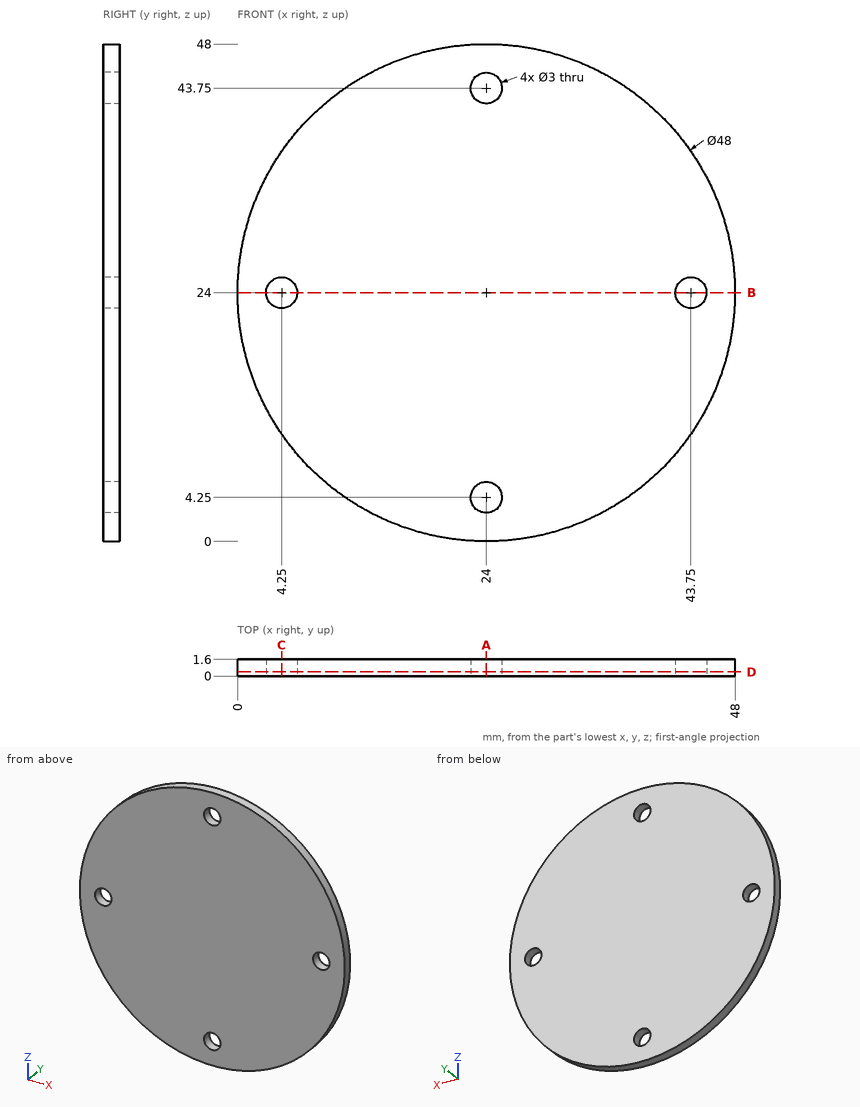
Source: three-view drawing plus pictorial views. Frame: mm from the lowest corner of the part. Round coordinates to 2 decimals unless told otherwise and drop trailing zeros. Write each loop counter-clockwise with the first axis right and the second up, starting at its lowest first coordinate (ties: lowest second). Pieces come first, ordered by that corner, then holes. Notation, with made-up numbers: M -29.5,-38 L 23.5,-38 A18 ccw 23.5,-24 Z; hole C 50,1.25 d2. An arc over 180 degrees is marked long. One line per item, written item: value. Start each with the question number.
Item 1: Section query D-D (y = 0.4). Return the cut outline in (x, z).
Item 2: Section query A-A (x = 24). Return the cut outline in (y, z), plus the area to 3 significant figures.
Item 3: Pin query (flat end, axial travel): pin 1 (2.5 mm diameter, centred on x = 24, z = 4.25, fed in from -Y). Return the tip coordinate at first contact, or that it passes through.
Item 4: Ray query, L1, parallel to X at y = 1.05, z = 24; L2, parallel to X at y = 0.7, z = 23; L3, parallel to Z at x = 45, y = 1.5. Return the intervals inside material, ascending. Write a range as from..to.
Item 5: Section query C-C (x = 4.25). Return the cut outline in (y, z), plus the area to 3 significant figures.
Item 6: Section query B-B (z = 24). Return the cut outline in (x, y), plus the area to 3 significant figures.
Result set:
1. outline: C 24,24 d48; hole C 4.25,24 d3; hole C 24,4.25 d3; hole C 24,43.75 d3; hole C 43.75,24 d3
2. outline: M 0,0 L 1.6,0 L 1.6,2.75 L 0,2.75 Z; M 0,5.75 L 1.6,5.75 L 1.6,42.25 L 0,42.25 Z; M 0,45.25 L 1.6,45.25 L 1.6,48 L 0,48 Z
2. area: 67.2 mm²
3. pin 1: passes through
4. L1: x = 0..2.75, 5.75..42.25, 45.25..48
4. L2: x = 0.02..3.13, 5.37..42.63, 44.87..47.98
4. L3: z = 12.38..23.17, 24.83..35.62
5. outline: M 0,10.36 L 1.6,10.36 L 1.6,22.5 L 0,22.5 Z; M 0,25.5 L 1.6,25.5 L 1.6,37.64 L 0,37.64 Z
5. area: 38.8 mm²
6. outline: M 0,0 L 2.75,0 L 2.75,1.6 L 0,1.6 Z; M 5.75,0 L 42.25,0 L 42.25,1.6 L 5.75,1.6 Z; M 45.25,0 L 48,0 L 48,1.6 L 45.25,1.6 Z
6. area: 67.2 mm²
